Geometry check sheet. Reference: the model listing, model coordinates, mm. A direction names the side the tool comes from. Give positions to 0.01 mm unless a question says otherwise; leave off trailing zeros. Loops run counter-clockwise (first coordinate to the right, second up) from the corner with the lowest first, then second, coordinate; pieces in that order, holes last. Notation, with made-up numbers: (-10, 70.5) -> (-3, 70.5) arc R26 cw to (-3, 107.5) -> close; hole circle Ø6 at (53.5, 45). An arc over 180 degrees is marked (long way). One line per question, with ' | ' between items.
from build123d import *

# Parameters (mm, degrees)
SKETCH_R     = 1.55
PAD_DEPTH    = 5.15
SKETCH001_W  = 26
SKETCH001_H  = 4.5
PAD001_DEPTH = 4.75


with BuildPart() as part:
    # Sketch → Pad (new body, symmetric)
    with BuildSketch(Plane.XY):
        with BuildLine():
            Line((-11.1, 7.95), (11.1, 7.95))
            ThreePointArc((13.9, 5.15), (13.079899, 7.129899), (11.1, 7.95))
            Line((13.9, 5.15), (13.9, -5.15))
            ThreePointArc((11.1, -7.95), (13.079899, -7.129899), (13.9, -5.15))
            Line((-11.1, -7.95), (11.1, -7.95))
            ThreePointArc((-13.9, -5.15), (-13.079899, -7.129899), (-11.1, -7.95))
            Line((-13.9, 5.15), (-13.9, -5.15))
            ThreePointArc((-11.1, 7.95), (-13.079899, 7.129899), (-13.9, 5.15))
        make_face()
        with Locations((-11.1, 5.15)):
            Circle(SKETCH_R, mode=Mode.SUBTRACT)
        with Locations((11.1, -5.15)):
            Circle(SKETCH_R, mode=Mode.SUBTRACT)
    extrude(amount=PAD_DEPTH, both=True)

    # Sketch001 → Pad001 (join, symmetric)
    with BuildSketch(Plane.XY):
        with BuildLine():
            Line((-2, 9.25), (51.9, 9.25))
            Line((51.9, 9.25), (51.9, 9.95))
            Line((51.9, 9.95), (-2.7, 9.95))
            ThreePointArc((-2.7, 9.95), (-2.912132, 9.862132), (-3, 9.65))
            Line((-3, 9.65), (-3, 7.95))
            Line((-3, 7.95), (-2.3, 7.95))
            Line((-2.3, 8.95), (-2.3, 7.95))
            ThreePointArc((-2, 9.25), (-2.212132, 9.162132), (-2.3, 8.95))
        make_face()
        with Locations((-26.9, -0.3)):
            Rectangle(SKETCH001_W, SKETCH001_H)
        with Locations((-26.9, -6.3)):
            Rectangle(SKETCH001_W, SKETCH001_H)
        Polygon((-28.9, -8.7), (-1.9, -8.7), (-1.9, -7.95), (-0.9, -7.95), (-0.9, -13.2), (-28.9, -13.2), align=None)
    extrude(amount=PAD001_DEPTH, both=True)


solid = part.part
Item 1: Set-up check for faces 1 (the face through (13.9, 0, 0)), 2 (the face through (-27, -6, -4.75)), 3 (the face through (-13, -8.7, 0)): record each of +Z, -Z, +X, -X, +Y, -Y from which the full face is reachable in a straight line by a thin tool's end or side.
Result:
face 1: +Z, -Z, +X, -Y | face 2: -Z, -X, +Y, -Y | face 3: +Z, -Z, -X
Item 2: Release check for a two-part mould opening along Y. For faces 4 (the face through (24.3, 9.7, -4.75)), 5 (the face through (-27, -2.55, 0)), 6 (the face through (25, 9.95, 0)) record: pulls with the +Y half, pulls with the -Y half, needs draft (parallel to the pull), parting line crosses it, or undercut.
Result:
face 4: needs draft | face 5: undercut | face 6: pulls with the +Y half
Item 3: Scan lines: probe 1 along Y at (x, z) = (11.1, 0.5); probe 2 along Y at (x, z) = (-11.1, 1); probe 3 along X at (y, z) = (3, 4). Record each from-to range of solid material in increasing order.
Result:
probe 1: -7.95 to -6.7, -3.6 to 7.95, 9.25 to 9.95 | probe 2: -13.2 to -8.7, -7.95 to 3.6, 6.7 to 7.95 | probe 3: -13.9 to 13.9
Item 4: Sectioned sample at A-A (z = 3.25). Give the number of separate pieces and of enclosed holes in the cut face, plus the area to 3 significant figures.
Result:
separate pieces: 1 | enclosed holes: 2 | area: 820 mm2
Item 5: Depth check by flat-ended pin: pin 1 Ø6 at (x, y) = (-15.5, -9.5) entering from +Z; pin 2 Ø2 at (y, z) = (-0.5, -3) entering from +X; pin 3 Ø3 at (x, z) = (-32, 0) entering from +Y. Enter the tip coordinate at first touch or a pass-through.
Result:
pin 1: z = 4.75 | pin 2: x = 13.9 | pin 3: y = 1.95
Item 6: Sectioned sample at C-C (x = 36.5). Record the cut outline in (y, z), plus the area to 3 significant figures.
Result:
outline: (9.25, -4.75) -> (9.95, -4.75) -> (9.95, 4.75) -> (9.25, 4.75) -> close | area: 6.65 mm2
Item 7: Sectioned sample at B-B (y = 0). Record the cut outline in (x, z).
Result:
outline: (-39.9, -4.75) -> (-13.9, -4.75) -> (-13.9, -5.15) -> (13.9, -5.15) -> (13.9, 5.15) -> (-13.9, 5.15) -> (-13.9, 4.75) -> (-39.9, 4.75) -> close
